```python
from build123d import *

# Parameters (mm, degrees)
BOSS_EXTRUDE1_DEPTH = 2.5
SKETCH2_R           = 1.7
CUT_EXTRUDE1_DEPTH  = 1.5
FILLET1_R           = 1.5


with BuildPart() as part:
    # Sketch1 → Boss-Extrude1 (new body)
    with BuildSketch(Plane.XY):
        Polygon((-7.56419618, 12.7), (-7.56419618, 9.2), (5.44580382, 0), (5.44580382, 12.7), align=None)
    extrude(amount=BOSS_EXTRUDE1_DEPTH)

    # Sketch2 → Cut-Extrude1 (cut)
    with BuildSketch(Plane.XY.offset(2.5)):
        with Locations((-4.31419618, 9.2)):
            Circle(SKETCH2_R)
    extrude(amount=-CUT_EXTRUDE1_DEPTH, mode=Mode.SUBTRACT)

    # Mirror2: part across plane


with BuildPart() as part_1:
    add(part.part)
    add(part.part.mirror(Plane(origin=(5.44580382, 0, 2.5), x_dir=(0, 0, 1), z_dir=(-1, 0, 0))))

    # Fillet1
    fillet1_edges = [part_1.edges().sort_by_distance(p)[0] for p in [
        (18.45580382, 12.7, 1.25),
        (18.45580382, 9.2, 1.25),
        (5.44580382, 0, 1.25),
        (18.45580382, 10.95, 0),
        (11.95080382, 4.6, 0),
        (-1.05919618, 4.6, 0),
        (-7.56419618, 10.95, 0),
        (5.44580382, 12.7, 0),
        (-7.56419618, 9.2, 1.25),
        (-7.56419618, 12.7, 1.25),
    ]]
    fillet(fillet1_edges, radius=FILLET1_R)


solid = part_1.part
```
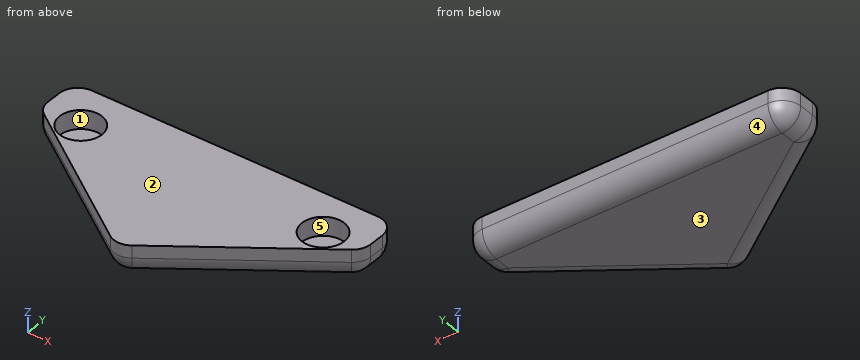
Geometry check sheet. Reference: the model listing, model coordinates, mm. Face numbers are marked on the shaded views. A direction names the side the tool comes from. Round coordinates to 2 decimals unless told otherwise and drop trailing zeros. Loops run counter-clockwise (first coordinate to the right, second up) from the corner with the lowest first, then second, coordinate; pieces in that order, holes last. Notation, with made-up numbers: (19.25, 22) - (27.25, 22) arc R29 ccw to (27.25, 52) - close; hole circle Ø4 at (78.25, -27). An arc over 180 degrees is marked (long way). Use a Markdown table: item, result.
Q1. Go/stop test with flat-tipped pins: P1, Ø5, axis at x = -3.5, y = 3.5, coming from the +Z side; P2, Ø3, axis at x = -4.31, y = 9.2, coming from the +Z side. Record where each tip stops, or that it passes through.
Solutions:
| item | result |
|---|---|
| P1 | stops at z = 2.5 |
| P2 | stops at z = 1 |
Q2. Draft check along Y on the marked faces 3, 4 and 5. Enter one of: released by +Y, released by -Y, zero draft, split by the parting line, or undercut.
Solutions:
| item | result |
|---|---|
| face 3 | zero draft |
| face 4 | released by +Y |
| face 5 | undercut |
Q3. Access from +Z, -Z, +X, -X, +Y, -Y to the whole of each face (thin tool, end or side, straight path). Record for the marked faces 1 and 2.
Solutions:
| item | result |
|---|---|
| face 1 | +Z |
| face 2 | +Z, +X, -X, +Y, -Y |
Q4. Material ranges on line 1 (X direction, y = 10, z = 1.35); line 2 (X direction, y = 9.5, z = 1.1); line 3 (Z direction, x = 14, y = 8.5), recorded low to high.
Solutions:
| item | result |
|---|---|
| line 1 | x = -7.56 to -5.81, -2.81 to 13.71, 16.71 to 18.45 |
| line 2 | x = -7.43 to -5.99, -2.64 to 13.53, 16.88 to 18.32 |
| line 3 | z = 0 to 1 |
Q5. Cross-section at A-A on z = 0.3. Record the cut outline in (x, y), plus the area to 3 significant figures.
Solutions:
| item | result |
|---|---|
| outline | (-6.96, 9.98) arc R0.9 ccw to (-6.58, 9.24) - (4.93, 1.1) arc R0.9 ccw to (5.97, 1.1) - (17.48, 9.24) arc R0.9 ccw to (17.86, 9.98) - (17.86, 11.2) arc R0.9 ccw to (16.96, 12.1) - (-6.06, 12.1) arc R0.9 ccw to (-6.96, 11.2) - close |
| area | 173 mm2 |
